from build123d import *

# Parameters (mm, degrees)
F1_DEPTH = 5
F3_DEPTH = 20
F5_D     = 5.5
F7_D     = 5
F9_D     = 5


with BuildPart() as f1:
    # F0 (on Front) → F1 (new body)
    with BuildSketch(Plane.XZ):
        Polygon((36, 0), (0, 0), (-36, 0), (-47.5470053838, -20), (0, -20), (47.5470053838, -20), align=None)
    extrude(amount=F1_DEPTH)

    # F2 (on face) → F3 (join)
    with BuildSketch(Plane.XZ.offset(5)):
        Polygon((-30.2264973081, 0), (-36, 0), (-47.5470053838, -20), (-41.7735026919, -20), (-33.1132486541, -5), align=None)
        Polygon((30.2264973081, 0), (-30.2264973081, 0), (-33.1132486541, -5), (33.1132486541, -5), align=None)
        Polygon((36, 0), (30.2264973081, 0), (33.1132486541, -5), (41.7735026919, -20), (47.5470053838, -20), align=None)
    extrude(amount=F3_DEPTH)

    # F5 (through all)
    with Locations(Plane.XZ.offset(5)):
        with Locations((0, -13.6782340705)):
            Hole(F5_D / 2)

    # F7 (through all)
    with Locations(Plane(origin=(27, 0, 15.5884572681), x_dir=(0, 1, 0), z_dir=(0.8660254038, 0, 0.5))):
        with Locations((-12.5, -29)):
            Hole(F7_D / 2)

    # F9 (through all)
    with Locations(Plane(origin=(-27, 0, 15.5884572681), x_dir=(0, -1, 0), z_dir=(-0.8660254038, 0, 0.5))):
        with Locations((12.5, -29)):
            Hole(F9_D / 2)


solid = f1.part
The listing builds one solid part. Answer for the finished solid, in the listing's coordinates (mm). A direction names the side the tool comes from. Give positions to 0.01 mm unless a question says otherwise; leave off trailing zeros. Loops run counter-clockwise (first coordinate to the right, second up) from the corner with the lowest first, then second, coordinate; pieces in that order, holes last.
Item 1: A cutting plane is placed at C-C (z = -15.25). Give the vertices of the cut face in (x, y), then the cut area to 3 significant figures.
Derived:
outline: (-44.8, -25) - (-39.03, -25) - (-39.03, -5) - (-2.26, -5) - (-2.26, 0) - (-44.8, 0) - close; (2.26, -5) - (39.03, -5) - (39.03, -25) - (44.8, -25) - (44.8, 0) - (2.26, 0) - close
area: 656 mm2
Item 2: A cutting plane is placed at A-A (x = 0). Give the vertices of the cut face in (y, z), then the cut area to 4 significant figures.
Derived:
outline: (-25, -5) - (-5, -5) - (-5, -10.93) - (0, -10.93) - (0, 0) - (-25, 0) - close; (-5, -20) - (0, -20) - (0, -16.43) - (-5, -16.43) - close
area: 172.5 mm2
Item 3: A cutting plane is placed at B-B (y = -14). Give the vertices of the cut face in (x, z).
Derived:
outline: (-47.55, -20) - (-41.77, -20) - (-38.17, -13.76) - (-42.5, -11.26) - close; (-40.5, -7.79) - (-36.17, -10.29) - (-33.11, -5) - (33.11, -5) - (36.17, -10.29) - (40.5, -7.79) - (36, 0) - (-36, 0) - close; (38.17, -13.76) - (41.77, -20) - (47.55, -20) - (42.5, -11.26) - close
Item 4: Determine the mould class of faces 1 (the flat face through (-42.976, -12.325, -12.082)), 2 (the flat face through (36.42, -14.86, -10.73)), 3 (the cylindrical face through (38.46, -10.66, -9.33)) for opening direction Z: +Z half, -Z half, draft (parallel to the pull), parting line (faces both ways), or undercut.
Derived:
face 1: +Z half
face 2: -Z half
face 3: undercut
Item 5: A cutting plane is placed at D-D (y = -7). Give the vertices of the cut face in (x, z).
Derived:
outline: (-47.55, -20) - (-41.77, -20) - (-33.11, -5) - (33.11, -5) - (41.77, -20) - (47.55, -20) - (36, 0) - (-36, 0) - close
Item 6: Each of these flat-tipped pins is pushed along its axis until it touches: pin 1 Ø1 at (x, z) = (32, -9) entering from -Y; pin 2 Ø8 at (y, z) = (-13.5, -10.5) entering from -X; pin 3 Ø3 at (y, z) = (-18, -12.5) entering from -X. Where does it stop, or does it pass through?
Derived:
pin 1: stops at y = -5
pin 2: stops at x = -44.37
pin 3: stops at x = -44.08
Item 7: A tool of negligible diameter and unlimited length cuts with its end or side. For faces 4 (the flat face through (0, -15, -5)), 5 (the flat face through (0, -4, -20)), from which of +Z, -Z, +X, -X, +Y, -Y can it reach the whole face along a straight path? Write none if from no direction.
Derived:
face 4: -Z, -Y
face 5: -Z, +X, -X, +Y, -Y
Item 8: Find the intervals of material crossed by line 1 along Z through (x, y) = (0, -2.5); line 2 along Y through (x, z) = (-35, -10), in increasing order.
Derived:
line 1: z = -20 to -16.43, -10.93 to 0
line 2: y = -5 to 0
